Here's how the part is built. I have some questions about the finished solid (model axes, mm). Face numbers are marked on the shaded views. A direction names the side the tool comes from. Give positions to 0.01 mm unless a question says otherwise; leave off trailing zeros. Order: outer loops, then holes, each group sorted by start corner. A loop starts at its lowest first (then second) coordinate and runs counter-clockwise, first axis right, second up. Notation, with made-up numbers: M 77.25,-5.5 L 103.25,-5.5 A22 ccw 103.25,2.5 Z; hole C 36.25,-17 d3. An arc over 180 degrees is marked long. Use one line per item in the form item = value.
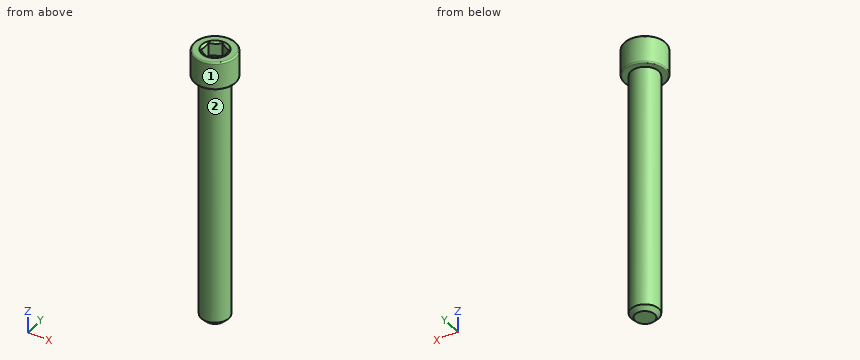
from build123d import *

# Parameters (mm, degrees)
CUT_EXTRUDE1_START = 31.75
CUT_EXTRUDE1_DEPTH = 3.175


with BuildPart() as part:
    # Sketch2 → Revolve1 (revolve)
    with BuildSketch(Plane(origin=(0, 0, 0), x_dir=(0, 0, -1), z_dir=(1, 0, 0)), mode=Mode.PRIVATE) as revolve1_sk:
        with BuildLine():
            Line((31.75, 0), (31.75, 2.2225))
            Line((31.75, 2.2225), (30.7975, 3.175))
            Line((30.7975, 3.175), (-25.4, 3.175))
            Line((-25.4, 3.175), (-25.4, 4.445))
            ThreePointArc((-25.4, 4.445), (-25.492993597, 4.669506403), (-25.7175, 4.7625))
            Line((-25.7175, 4.7625), (-31.4325, 4.7625))
            ThreePointArc((-31.4325, 4.7625), (-31.657006403, 4.669506403), (-31.75, 4.445))
            Line((-31.75, 4.445), (-31.75, 0))
            Line((-31.75, 0), (31.75, 0))
        make_face()
    revolve(revolve1_sk.sketch.rotate(Axis((0, 0, -31.75), (0, 0, 1)), 90), axis=Axis((0, 0, -31.75), (0, 0, 1)))

    # Sketch3 → Cut-Extrude1 (cut)
    with BuildSketch(Plane.XY.offset(CUT_EXTRUDE1_START)):
        Polygon((-2.38125, 1.374815329), (-2.38125, -1.374815329), (0, -2.749630657), (2.38125, -1.374815329), (2.38125, 1.374815329), (0, 2.749630657), align=None)
    extrude(amount=-CUT_EXTRUDE1_DEPTH, mode=Mode.SUBTRACT)

    # Cut-Extrude2 cone 1 section (through the dimple's axis) → Cut-Extrude2 (revolve, cut)
    with BuildSketch(Plane(origin=(0, 0, 31.75), x_dir=(0, -1, 0), z_dir=(1, 0, 0))):
        Polygon((0, 0), (3.032192214, 0), (0, 1.750636991), align=None)
    revolve(axis=Axis((0, 0, 31.75), (0, 0, -1)), mode=Mode.SUBTRACT)


solid = part.part
Q1. I want a section at B-B on z = -25. Write out the boundary of the cut face in (x, y) (3 decimals).
Found:
outline = C 0,0 d6.35
Q2. I need wall thicknesses on L1, parallel to X at y = -0.25, z = -22.5; L2, parallel to Y at x = 0, z = 1 (3 decimals); L3, parallel to Z at x = 2.75, y = 2.25. Which ranges of each line are inside material? Lowest first, please.
Found:
L1 = -3.17 to 3.17
L2 = -3.175 to 3.175
L3 = 25.4 to 31.75
Q3. On a 3-axis mill with a long thin cutter (end or side, diameter ignored), from which of +Z, -Z, +X, -X, +Y, -Y can I reach the whole of each face in a straight line? I mean the marked faces 1 and 2. Say none if no direction works.
Found:
face_1 = +Z, -Z
face_2 = -Z
Q4. I'm going to push flat-ended pins straight in: pin 1 Ø2 at (x, z) = (-3, -14.5) entering from -Y; pin 2 Ø1.5 at (x, y) = (0, 3.5) entering from -Z; pin 3 Ø1.5 at (x, y) = (0.5, 2) entering from +Z. Where does each tip first touch, or does it pass through?
Found:
pin_1 = -2.47
pin_2 = -31.22
pin_3 = 31.62
